Design review of the part built by this model. Coordinates are the model's own, in mm. A direction names the side the tool comes from. Round coordinates to 2 decimals unless told otherwise and drop trailing zeros. Order: outer loops, then holes, each group sorted by start corner. A loop starts at its lowest first (then second) coordinate and runs counter-clockwise, first axis right, second up. Notation, with made-up numbers: (89.25, -10.5) - (124.25, -10.5) arc R17 ccw to (124.25, -6.5) - close; hole circle Ø3 at (66, 28.25). An arc over 180 degrees is marked (long way). Use CSV: the item, a comma, the result in double quotes.
from build123d import *

# Parameters (mm, degrees)
SKETCH1_W                      = 15.24
SKETCH1_H                      = 20.32
BOSS_EXTRUDE1_DEPTH            = 1.5875
SKETCH2_W                      = 2.54
SKETCH2_H                      = 20.32
F_1_16_0_0625_DIAMETER_HOLE1_D = 1.5875
SKETCH10_W                     = 5.245479694
SKETCH10_H                     = 5.08
CUT_EXTRUDE1_DEPTH             = 6.35


with BuildPart() as part:
    # Sketch1 → Boss-Extrude1 (new body)
    with BuildSketch(Plane.XY):
        Rectangle(SKETCH1_W, SKETCH1_H)
    extrude(amount=BOSS_EXTRUDE1_DEPTH)

    # Sketch2 → Revolve-Thin1 (revolve)
    with BuildSketch(Plane(origin=(7.62, 0, 0), x_dir=(0, 0, -1), z_dir=(1, 0, 0))):
        with Locations((-2.06375, 0)):
            Rectangle(SKETCH2_W, SKETCH2_H)
    revolve(axis=Axis((7.62, -10.16, 0.79375), (0, 1, 0)))

    # 1/16 (0.0625) Diameter Hole1 (through all)
    with Locations(Plane(origin=(0, 10.16, 0), x_dir=(1, 0, 0), z_dir=(0, 1, 0))):
        with Locations((7.62, -1.27)):
            Hole(F_1_16_0_0625_DIAMETER_HOLE1_D / 2)

    # Sketch10 → Cut-Extrude1 (cut, symmetric)
    with BuildSketch(Plane.XY.offset(1.5875)):
        with Locations((7.960094746, 2.54)):
            Rectangle(SKETCH10_W, SKETCH10_H)
        with Locations((7.960094746, -7.62)):
            Rectangle(SKETCH10_W, SKETCH10_H)
    extrude(amount=CUT_EXTRUDE1_DEPTH, both=True, mode=Mode.SUBTRACT)


solid = part.part
1) Insertion check: pin 1 Ø1.4 at (x, z) = (8.5, 0.5) entering from -Y; pin 2 Ø3 at (x, z) = (-2, -1) entering from +Y; pin 3 Ø1.1 at (y, z) = (2.5, 1) entering from +X; pin 4 Ø10.5 at (x, y) = (-2.5, -3.5) entering from +Z. Each pin has a flat end and moves straight along its axis. Give the tip position at first contact, or say it passes through.
Data:
pin 1,"stops at y = -5.08"
pin 2,"stops at y = 10.16"
pin 3,"stops at x = 5.34"
pin 4,"stops at z = 1.59"
2) We need section B-B (y = -3). Give the boundary of the cut face in (x, z), then the cut area to 3 significant figures.
Data:
outline,"(-7.62, 0) - (5.21, 0) arc R2.54 ccw (long way) to (5.21, 1.59) - (-7.62, 1.59) - close; hole circle Ø1.59 at (7.62, 1.27)"
area,"38.5 mm2"
3) For faces 5 (the face through (-1, 0, 0)), 6 (the face through (-1, 0, 1.588)), 7 (the face through (5.337, -8, 1)), 8 (the face through (10.16, 6.92, 0.89)), 9 (the face through (8, 0, 0)), list the 3-axis set-ups (+Z, -Z, +X, -X, +Y, -Y) from which the entire face can be reached by the end or side of a thin tool; tool diameter is ignored.
Data:
face 5,"-Z, -X, +Y, -Y"
face 6,"+Z, -X, +Y, -Y"
face 7,"+Z, -Z, +X, -Y"
face 8,"+Y, -Y"
face 9,"+Z, -Z, +X"
4) We need section A-A (x = 7.62). Give the boundary of the cut face in (y, z).
Data:
outline,"(-5.08, -1.75) - (0, -1.75) - (0, 0.48) - (-5.08, 0.48) - close; (-5.08, 2.06) - (0, 2.06) - (0, 3.33) - (-5.08, 3.33) - close; (5.08, -1.75) - (10.16, -1.75) - (10.16, 0.48) - (5.08, 0.48) - close; (5.08, 2.06) - (10.16, 2.06) - (10.16, 3.33) - (5.08, 3.33) - close"
5) The part is to be moulded in two halves that separate along X. For faces 1 (the face through (8.413, -2.576, 1.235)), 2 (the face through (8.413, 7.584, 1.235)), 3 (the face through (-7.62, 0, 1)), 4 (the face through (8, 5.08, 0)), say which applies: +X half, -X half, draft (parallel to the pull), parting line (faces both ways), or undercut.
Data:
face 1,"undercut"
face 2,"undercut"
face 3,"-X half"
face 4,"draft"
6) We need section D-D (y = 3.5). Give the boundary of the cut face in (x, z).
Data:
outline,"(-7.62, 0) - (5.21, 0) arc R2.54 ccw to (5.34, -0.32) - (5.34, 1.91) arc R2.54 ccw to (5.21, 1.59) - (-7.62, 1.59) - close"
7) We need section C-C (z = 2.5). Give the boundary of the cut face in (x, y), then the cut area to 3 significant figures.
Data:
outline,"(5.74, -5.08) - (9.5, -5.08) - (9.5, 0) - (5.74, 0) - close; (5.74, 5.08) - (9.5, 5.08) - (9.5, 10.16) - (5.74, 10.16) - close"
area,"38.2 mm2"
8) To check wall thickness, follow L1, parallel to Y at x = 5.75, z = -0.8; L2, parallel to Z at x = 7.62, y = 6.1; L3, parallel to Z at x = 1.75, y = 3. State the ranges of each line that lie inside material, in increasing order. Write a range as from..to.
Data:
L1,"y = -5.08..0, 5.08..10.16"
L2,"z = -1.75..0.48, 2.06..3.33"
L3,"z = 0..1.59"
